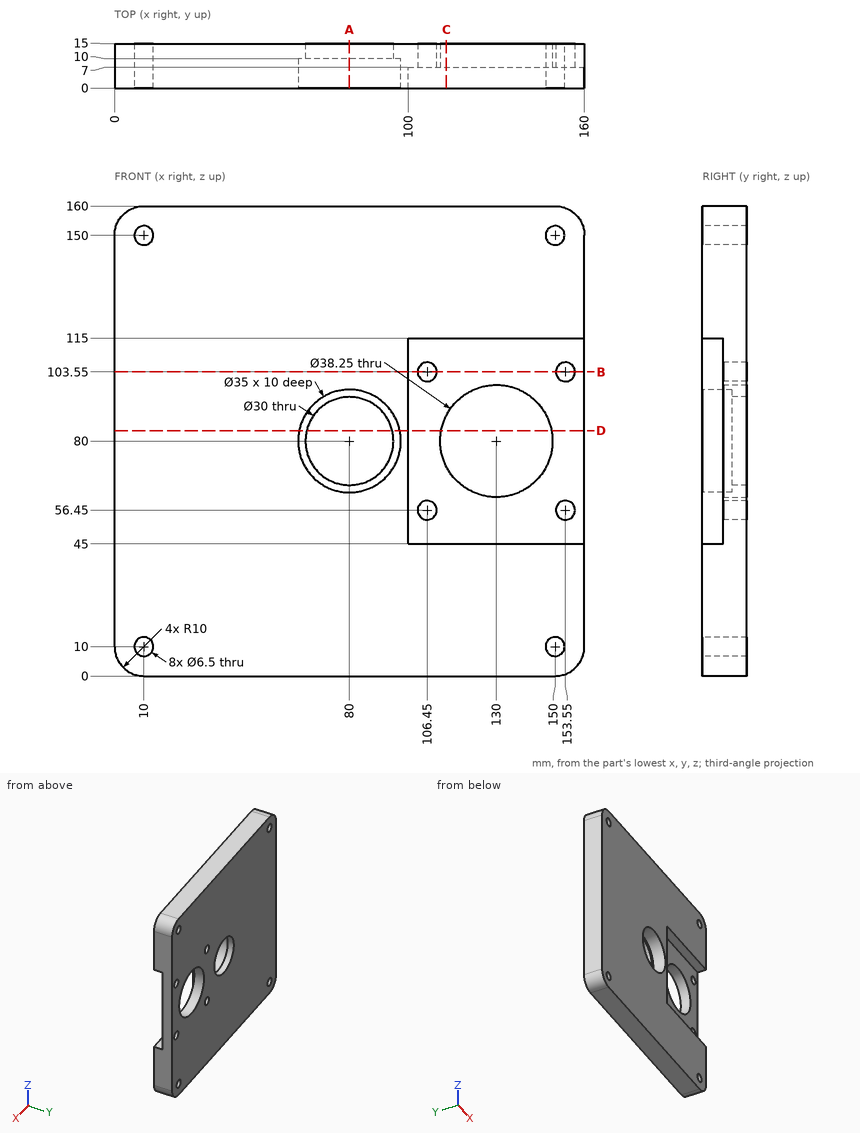
Geometry check sheet. Reference: drawing and pictorial views, mm from the part's lowest x, y, z. Give positions to 0.01 mm unless a question says otherwise; leave off trailing zeros. Loops run counter-clockwise (first coordinate to the right, second up) from the corner with the lowest first, then second, coordinate; pieces in that order, holes last.
1. Section check C-C, the plane x = 113. Enter the section's corners in (y, z), then the cut area to 3 significant figures.
2. Thickness scan on line 1 (Z direction, x = 10, y = 7.5); line 2 (Z direction, x = 106.45, y = 11). Record the ranges inside material, lowest first.
3. Section check A-A, the plane x = 80. Enter the section's corners in (y, z), then the cut area to 3 significant figures.
4. Section check D-D, the plane z = 83.5. Enter the section's corners in (x, y).
5. Section check B-B, the plane z = 103.55. Enter the section's corners in (x, y).
6. Go/stop test with flat-tipped pins: pin 1 Ø21 at (x, z) = (80, 80) entering from -Y; pin 2 Ø6 at (y, z) = (13.5, 109.5) entering from -X; pin 3 Ø10.5 at (x, z) = (106.45, 103.55) entering from -Y; pin 4 Ø7.5 at (y, z) = (2.5, 66.5) entering from +X. Record where each tip stops, or that it passes through.
Geometry says:
1. outline: (0, 0) - (15, 0) - (15, 71.24) - (7, 71.24) - (7, 45) - (0, 45) - close; (0, 115) - (7, 115) - (7, 88.76) - (15, 88.76) - (15, 160) - (0, 160) - close
1. area: 1,770 mm2
2. line 1: z = 0 to 6.75, 13.25 to 146.75, 153.25 to 160
2. line 2: z = 0 to 53.2, 59.7 to 100.3, 106.8 to 160
3. outline: (0, 0) - (15, 0) - (15, 65) - (10, 65) - (10, 62.5) - (0, 62.5) - close; (0, 97.5) - (10, 97.5) - (10, 95) - (15, 95) - (15, 160) - (0, 160) - close
3. area: 1,900 mm2
4. outline: (0, 0) - (62.85, 0) - (62.85, 10) - (65.41, 10) - (65.41, 15) - (0, 15) - close; (94.59, 10) - (97.15, 10) - (97.15, 0) - (100, 0) - (100, 7) - (111.2, 7) - (111.2, 15) - (94.59, 15) - close; (148.8, 7) - (160, 7) - (160, 15) - (148.8, 15) - close
5. outline: (0, 0) - (100, 0) - (100, 7) - (103.2, 7) - (103.2, 15) - (0, 15) - close; (109.7, 7) - (150.3, 7) - (150.3, 15) - (109.7, 15) - close; (156.8, 7) - (160, 7) - (160, 15) - (156.8, 15) - close
6. pin 1: passes through
6. pin 2: stops at x = 0
6. pin 3: stops at y = 7
6. pin 4: stops at x = 100
